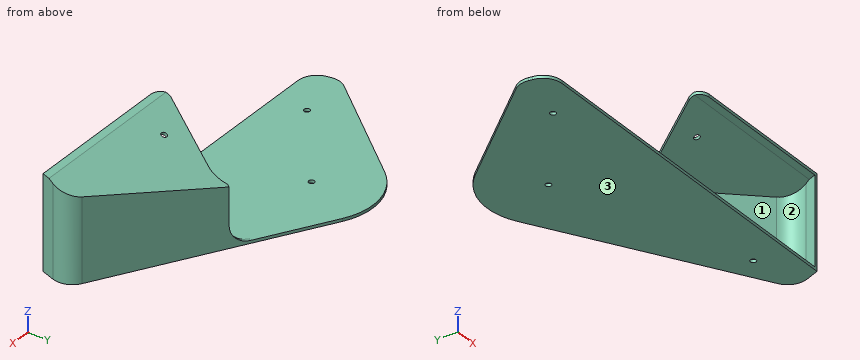
```python
from build123d import *

# Parameters (mm, degrees)
SKETCH_1_R          = 1.5
EXTRUDE_1_DEPTH     = 46
SKETCH_6_W          = 244.099615043
SKETCH_6_H          = 133.346377704
CUT_EXTRUDE_3_DEPTH = 339.792470358
SHELL_1_T           = 1.5
CUT_EXTRUDE_START   = -1.5
CUT_EXTRUDE_2_DEPTH = 342.316954288
FILLET_2_R          = 10
FILLET_3_R          = 10
FILLET_4_R          = 5
SKETCH_7_W          = 1.712142643
SKETCH_7_H          = 34.810742179
CUT_EXTRUDE_4_DEPTH = 5
FILLET_5_R          = 10
SKETCH_10_R         = 1.5
CUT_EXTRUDE_5_DEPTH = 2
SKETCH_11_R         = 1.5
CUT_EXTRUDE_6_DEPTH = 2


with BuildPart() as part:
    # 草图1 → 凸台-拉伸1 (new body)
    with BuildSketch(Plane.XY):
        with BuildLine():
            Line((-186.419017908, -172.076823512), (-234.49796572, -229.375082296))
            Line((-234.49796572, -229.375082296), (-231.975297342, -243.681845608))
            Line((-231.975297342, -243.681845608), (-41.975297342, -243.681845608))
            Line((-41.975297342, -243.681845608), (-36.768061348, -229.375082296))
            Line((-36.768061348, -229.375082296), (-147.804662393, -165.268070792))
            ThreePointArc((-147.804662393, -165.268070792), (-168.350931812, -161.645209141), (-186.419017908, -172.076823512))
        make_face()
        with Locations((-163.054662393, -191.681845608)):
            Circle(SKETCH_1_R, mode=Mode.SUBTRACT)
    extrude(amount=EXTRUDE_1_DEPTH)

    # 草图6 → 切除-拉伸3 (cut, through all)
    with BuildSketch(Plane(origin=(0, -13.84451284, -37.461622979), x_dir=(1, 0, 0), z_dir=(0, 0.3466501408716292, 0.9379944988291136))):
        with Locations((-134.599820809, -204.098171804)):
            Rectangle(SKETCH_6_W, SKETCH_6_H)
    extrude(amount=CUT_EXTRUDE_3_DEPTH, mode=Mode.SUBTRACT)

    # 抽壳1
    shell_1_openings = [part.faces().sort_by_distance(p)[0] for p in [
        (-136.975297342, -243.681845608, 23),
        (-164.554662393, -191.681845608, 14.463541988),
    ]]
    offset(amount=SHELL_1_T, openings=shell_1_openings, kind=Kind.INTERSECTION)

    # 草图2 → 切除-拉伸2 (cut, through all)
    with BuildSketch(Plane(origin=(0, 0, -1.5), x_dir=(-1, 0, 0), z_dir=(0, 0, -1)).offset(CUT_EXTRUDE_START)):
        with BuildLine():
            Line((103.691214377, -202.861337532), (127.258945703, -243.681845608))
            Line((127.258945703, -243.681845608), (233.49843726, -243.681845608))
            Line((233.49843726, -243.681845608), (236.096637562, -228.946719467))
            Line((236.096637562, -228.946719467), (187.568084573, -171.112642098))
            ThreePointArc((187.568084573, -171.112642098), (168.611404078, -160.167997512), (147.054662393, -163.969032687))
            Line((147.054662393, -163.969032687), (102.8873668, -189.469032687))
            ThreePointArc((102.8873668, -189.469032687), (101.708543429, -196.260066445), (103.691214377, -202.861337532))
        make_face()
    extrude(amount=-CUT_EXTRUDE_2_DEPTH, mode=Mode.SUBTRACT)

    # 圆角2
    fillet_2_edges = [part.edges().sort_by_distance(p)[0] for p in [
        (-34.928038952, -228.705368914, 21.021316252),
        (-36.768061348, -229.375082296, 21.095489388),
    ]]
    fillet(fillet_2_edges, radius=FILLET_2_R)

    # 圆角3
    fillet_3_edges = [part.edges().sort_by_distance(p)[0] for p in [
        (-236.096637562, -228.946719467, -0.75),
        (-233.49843726, -243.681845608, -0.75),
    ]]
    fillet(fillet_3_edges, radius=FILLET_3_R)

    # 圆角4
    fillet_4_edges = [part.edges().sort_by_distance(p)[0] for p in [
        (-127.258945703, -243.681845608, 46.75),
    ]]
    fillet(fillet_4_edges, radius=FILLET_4_R)

    # 草图7 → 切除-拉伸4 (cut)
    with BuildSketch(Plane(origin=(-107.764339469, -186.653311204, 0), x_dir=(0.8660254037844399, -0.4999999999999979, 0), z_dir=(0.49999999999999784, 0.8660254037844398, 0))):
        with Locations((6.487514288, -17.40537109)):
            Rectangle(SKETCH_7_W, SKETCH_7_H)
    extrude(amount=-CUT_EXTRUDE_4_DEPTH, mode=Mode.SUBTRACT)

    # 圆角5
    fillet_5_edges = [part.edges().sort_by_distance(p)[0] for p in [
        (-101.779607776, -190.974623061, 0),
    ]]
    fillet(fillet_5_edges, radius=FILLET_5_R)

    # 草图10 → 切除-拉伸5 (cut)
    with BuildSketch(Plane(origin=(0, 0, -1.5), x_dir=(-1, 0, 0), z_dir=(0, 0, -1))):
        with Locations((208.054662393, -226.681845608)):
            Circle(SKETCH_10_R)
        with Locations((63.054662393, -226.681845608)):
            Circle(SKETCH_10_R)
    extrude(amount=-CUT_EXTRUDE_5_DEPTH, mode=Mode.SUBTRACT)

    # 草图11 → 切除-拉伸6 (cut)
    with BuildSketch(Plane(origin=(0, -13.324537629, -36.054631231), x_dir=(1, 0, 0), z_dir=(0, 0.3466501408716292, 0.9379944988291135))):
        with Locations(Location((-102.379030683, -225.76615913, 0), (0, 0, 270))):
            Circle(SKETCH_11_R)
    extrude(amount=-CUT_EXTRUDE_6_DEPTH, mode=Mode.SUBTRACT)


solid = part.part
```
Work out the finished part from the listing and answer in its coordinate system (mm). Face numbers are marked on the shaded views. A direction names the side the tool comes from. Give positions to 0.01 mm unless a question says otherwise; leave off trailing zeros. Write each loop counter-clockwise with the first axis right and the second up, starting at its lowest first coordinate (ties: lowest second). Pieces come first, ordered by that corner, then holes. Notation, with made-up numbers: (21.25, 55) - (53.25, 55) arc R22 ccw to (53.25, 86) - close; hole circle Ø5 at (-9.5, 54.5). An arc over 180 degrees is marked (long way). Use one line per item in the form item = value.
1. A cutting plane is placed at C-C (x = -76). Write down the section's boundary in (y, z).
Filled in:
outline = (-243.68, -1.5) - (-204.99, -1.5) - (-204.99, 34.78) - (-239.41, 47.5) - (-243.68, 47.5) - (-243.68, 46) - (-239.68, 46) - (-206.72, 33.82) - (-206.72, 0) - (-243.68, 0) - close
2. A cutting plane is placed at B-B (y = -211.5). Write down the section's boundary in (x, z), and give its area (3 significant figures).
Filled in:
outline = (-221.46, -1.5) - (-64.73, -1.5) - (-64.73, 37.18) - (-108.68, 37.18) - (-108.68, 35.58) - (-67.73, 35.58) - (-67.73, 0) - (-221.46, 0) - close
area = 412 mm^2
3. For the marked faces 1, 2 and 3, determine the directions among +Z, -Z, +X, -X, +Y, -Y from which every point of the face is accessible in a straight line to the end or side of a thin tool.
Filled in:
face_1 = -X, -Y
face_2 = -X
face_3 = -Z, +X, -X, +Y, -Y
4. A cutting plane is placed at D-D (x = -141). Write down the section's boundary in (y, z).
Filled in:
outline = (-243.68, -1.5) - (-167.46, -1.5) - (-167.46, 0) - (-243.68, 0) - close
5. Each of these flat-tipped pins is pushed along its axis until it touches: pin 1 Ø12 at (x, y) = (-146, -210.5) entering from +Z; pin 2 Ø3.5 at (x, y) = (-63.05, -226.68) entering from +Z; pin 3 Ø6 at (y, z) = (-197, 14) entering from -X. Where does it stop, or does it pass through?
Filled in:
pin_1 = 0
pin_2 = 43.44
pin_3 = -98.04
6. A cutting plane is placed at A-A (z = 21.5). Write down the section's boundary in (x, y).
Filled in:
outline = (-102.15, -191.62) - (-44.03, -225.18) arc R10 cw to (-39.64, -237.26) - (-41.98, -243.68) - (-40.38, -243.68) - (-37.8, -236.59) arc R10 ccw to (-42.19, -224.51) - (-101.4, -190.33) - close
7. Consider L1, parallel to Z at x = -117.5, y = -214.5; L2, parallel to Z at x = -83, y = -212.5; L3, parallel to Z at x = -78.5, y = -223.5. Determine where each line is inside the solid, lowest interval first.
Filled in:
L1 = -1.5 to 0
L2 = -1.5 to 0, 35.95 to 37.55
L3 = -1.5 to 0, 40.02 to 41.62
